```python
from build123d import *

# Parameters (mm, degrees)
F0_R            = 55.88
F0_R_2          = 23.622
F1_DEPTH        = 2.286
F0_R_3          = 59.055
F2_DEPTH        = 5.08
F0_R_4          = 62.23
F3_DEPTH        = 33.02
F4_R            = 3.175
F5_DEPTH        = 25.4
F5_COPIES_COUNT = 3
F7_R            = 34.1580603644
F7_R_2          = 3.175
F7_R_3          = 23.622
F8_DEPTH        = 1.524


# Not quite as in the source:
# - a pattern or mirror of a feature is missing from the dataset's text; its kind, count and spacing are read off the source's solid


with BuildPart() as f1:
    # F0 (on Top) → F1 (new body, symmetric)
    with BuildSketch(Plane.XY):
        Circle(F0_R)
        Circle(F0_R_2, mode=Mode.SUBTRACT)
    extrude(amount=F1_DEPTH, both=True)

    # F0 (on Top) → F2 (join)
    with BuildSketch(Plane.XY):
        Circle(F0_R_3)
        Circle(F0_R, mode=Mode.SUBTRACT)
    extrude(amount=-F2_DEPTH)

    # F0 (on Top) → F3 (join)
    with BuildSketch(Plane.XY):
        Circle(F0_R_4)
        Circle(F0_R_3, mode=Mode.SUBTRACT)
    extrude(amount=-F3_DEPTH)

    # F4 (on face) → F5 (cut)
    with BuildSketch(Plane.XY.offset(2.286)):
        with Locations((0, 28.702)):
            Circle(F4_R)
    f5 = extrude(amount=-F5_DEPTH, mode=Mode.SUBTRACT)

    # F5_copies: F5 ×3 about axis
    f5_copies_axis = Axis((0, 0, 0), (0, 0, 1))
    for i in range(1, F5_COPIES_COUNT):
        add(f5.rotate(f5_copies_axis, i * 360 / F5_COPIES_COUNT), mode=Mode.SUBTRACT)

    # F7 (on face) → F8 (cut)
    with BuildSketch(Plane(origin=(0, 0, -2.286), x_dir=(1, 0, 0), z_dir=(0, 0, -1))):
        Circle(F7_R)
        with Locations((0, -28.702)):
            Circle(F7_R_2, mode=Mode.SUBTRACT)
        Circle(F7_R_3, mode=Mode.SUBTRACT)
        with Locations((-24.8566611394, 14.351)):
            Circle(F7_R_2, mode=Mode.SUBTRACT)
        with Locations((24.8566611394, 14.351)):
            Circle(F7_R_2, mode=Mode.SUBTRACT)
    extrude(amount=-F8_DEPTH, mode=Mode.SUBTRACT)


solid = f1.part
```
CAD build for the part. Positions are in the model's coordinates, mm. A direction names the side the tool comes from. Round coordinates to 2 decimals unless told otherwise and drop trailing zeros. Loops run counter-clockwise (first coordinate to the right, second up) from the corner with the lowest first, then second, coordinate; pieces in that order, holes last. Notation, with made-up numbers: M -20.75,59.5 L 37.25,59.5 A18 cw 37.25,72.5 Z; hole C 60,49 d1. An arc over 180 degrees is marked long. Return JSON: item names as keys, results as strings. Group by question number.
(1) Mould opens along Y. For faces 1 (the cylindrical face through (24.17, -17.45, 0.78)), 2 (the cylindrical face through (-13.49, -60.75, -16.28)), 3 (the flat face through (-51, 23.3, 0)) say: +Y half, -Y half, draft (parallel to the pull), parting line (faces both ways), or undercut.
(2) Saw through at A-A, the plane x = 0. List the corners of the cut face in (y, z) (3 decimals), and give its area (3 significant figures).
(3) Tool access for faces 4 (the cylindrical face through (-7.3, 55.4, 1.2)), 5 (the flat face through (24, 1, 2.286)), 6 (the flat face through (22, -52, -5.08)): list every direction of +Z, -Z, +X, -X, +Y, -Y with a clear straight run to the whole face (end or side of a thin tool).
(4) Drop flat-ended pins along their axis: P1, Ø8, axis at y = -8, z = -4, coming from the -X side; P2, Ø3, axis at x = 2.5, y = 35.5, coming from the -Z side; P3, Ø5, axis at x = -24.86, y = -14.35, coming from the -Z side; P4, Ø2, axis at x = -6, z = -26.5, coming from the -Y side. Give the stop position or say it passes through.
(5) Saw through at C-C, the plane y = 15. List the corners of the cut face in (x, z), and give its area (3 significant figures).
(6) Wall check: probe 1 along Y at (x, z) = (0, -1); probe 2 along Y at (x, z) = (0, -4.1); probe 3 along Z at (x, y) = (-39.5, -32). Give the ranges that are in metal, low to high. Write a range as [from, to].
(7) Saw through at B-B, the plane y = 0. List the corners of the cut face in (x, z) (3 decimals), and give its area (3 significant figures).
(8) Saw through at D-D, the plane x = -50. List the corners of the cut face in (y, z), and give its area (3 significant figures).
Answer list:
{
 "1": {"face 1": "undercut", "face 2": "parting line", "face 3": "draft"},
 "2": {"outline": "M -62.23,-33.02 L -59.055,-33.02 L -59.055,-5.08 L -55.88,-5.08 L -55.88,-2.286 L -34.158,-2.286 L -34.158,-0.762 L -23.622,-0.762 L -23.622,2.286 L -55.88,2.286 L -55.88,0 L -62.23,0 Z; M 23.622,-0.762 L 25.527,-0.762 L 25.527,2.286 L 23.622,2.286 Z; M 31.877,-0.762 L 34.158,-0.762 L 34.158,-2.286 L 55.88,-2.286 L 55.88,-5.08 L 59.055,-5.08 L 59.055,-33.02 L 62.23,-33.02 L 62.23,0 L 55.88,0 L 55.88,2.286 L 31.877,2.286 Z", "area": "485 mm2"},
 "3": {"face 4": "+Z", "face 5": "+Z, +X, -X, +Y, -Y", "face 6": "-Z"},
 "4": {"P1": "x = -62.1", "P2": "z = -2.29", "P3": "through", "P4": "y = -62.03"},
 "5": {"outline": "M -60.4,-33.02 L -57.12,-33.02 L -57.12,-5.08 L -53.83,-5.08 L -53.83,-2.29 L -30.69,-2.29 L -30.69,-0.76 L -18.25,-0.76 L -18.25,2.29 L -53.83,2.29 L -53.83,0 L -60.4,0 Z; M 18.25,-0.76 L 30.69,-0.76 L 30.69,-2.29 L 53.83,-2.29 L 53.83,-5.08 L 57.12,-5.08 L 57.12,-33.02 L 60.4,-33.02 L 60.4,0 L 53.83,0 L 53.83,2.29 L 18.25,2.29 Z", "area": "537 mm2"},
 "6": {"probe 1": "[-62.23, -34.16], [34.16, 62.23]", "probe 2": "[-62.23, -55.88], [55.88, 62.23]", "probe 3": "[-2.29, 2.29]"},
 "7": {"outline": "M -62.23,-33.02 L -59.055,-33.02 L -59.055,-5.08 L -55.88,-5.08 L -55.88,-2.286 L -34.158,-2.286 L -34.158,-0.762 L -23.622,-0.762 L -23.622,2.286 L -55.88,2.286 L -55.88,0 L -62.23,0 Z; M 23.622,-0.762 L 34.158,-0.762 L 34.158,-2.286 L 55.88,-2.286 L 55.88,-5.08 L 59.055,-5.08 L 59.055,-33.02 L 62.23,-33.02 L 62.23,0 L 55.88,0 L 55.88,2.286 L 23.622,2.286 Z", "area": "505 mm2"},
 "8": {"outline": "M -37.05,-33.02 L -31.42,-33.02 L -31.42,-5.08 L -24.95,-5.08 L -24.95,-2.29 L 24.95,-2.29 L 24.95,-5.08 L 31.42,-5.08 L 31.42,-33.02 L 37.05,-33.02 L 37.05,0 L 24.95,0 L 24.95,2.29 L -24.95,2.29 L -24.95,0 L -37.05,0 Z", "area": "665 mm2"}
}
